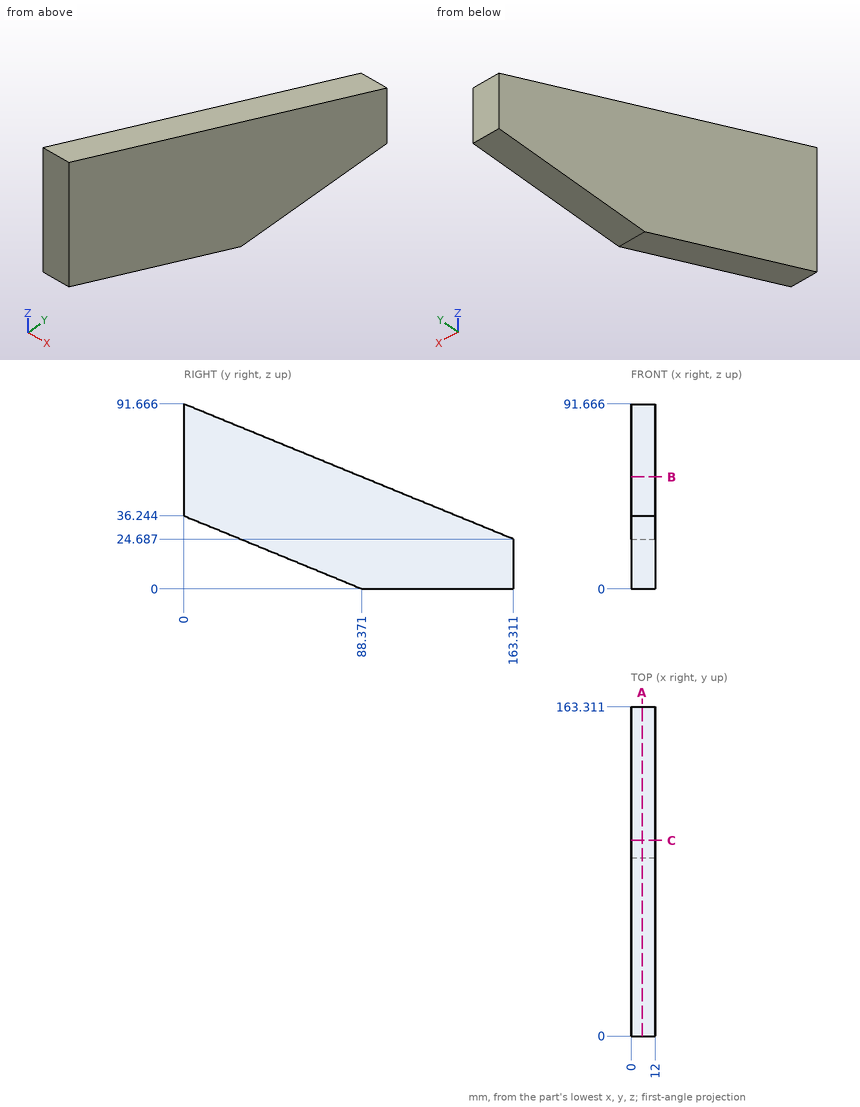
Answer from the drawing. Dimensions are ordinates in mm from the lowest x, y and z of the part. Give positions to 0.01 mm unless a question says otherwise; leave off trailing zeros. Order: outer loops, then holes, each group sorted by start corner. A loop starts at its lowest first (then second) coordinate and runs counter-clockwise, first axis right, second up. Notation, with made-up numbers: (60.25, 29) - (68.25, 29) arc R25 cw to (68.25, 64) - close; hole circle Ø7 at (17, 31.5). An arc over 180 degrees is marked (long way). One line per item, written item: value. Start each with the question number.
1) A cutting plane is placed at C-C on y = 97. Give the vertices of the cut face in (x, z).
2) A cutting plane is placed at B-B on z = 55.5. Give the vertices of the cut face in (x, y), then the cut area to 3 significant figures.
3) Find the intervals of material crossed by L1, parallel to Y at x = 10.5, z = 9.5 (1 decimal); L2, parallel to Z at x = 1, y = 82.5; L3, parallel to Z at x = 11, y = 80 (1 decimal), in increasing order.
4) Given pin 1 Ø6 at (x, y) = (2, 133.5) entering from +Z; pin 2 Ø1 at (x, z) = (3.5, 45) entering from +Y (1 decimal); pin 3 Ø1.5 at (x, z) = (2, 33) entering from +Y, each flat-ended and moving along its own axis, determine where each tip first touches the part or whether it passes through.
5) A cutting plane is placed at A-A on x = 5.5. Give the vertices of the cut face in (y, z) (1 decimal), then the cut area to 3 significant figures.
Answer sheet:
1. outline: (0, 0) - (12, 0) - (12, 51.88) - (0, 51.88) - close
2. outline: (0, 0) - (12, 0) - (12, 88.18) - (0, 88.18) - close
2. area: 1,060 mm2
3. L1: y = 65.2 to 163.3
3. L2: z = 2.41 to 57.83
3. L3: z = 3.4 to 58.9
4. pin 1: stops at z = 38.14
4. pin 2: stops at y = 115
4. pin 3: stops at y = 144.87
5. outline: (0, 36.2) - (88.4, 0) - (163.3, 0) - (163.3, 24.7) - (0, 91.7) - close
5. area: 7,900 mm2
